Read the model definition and answer for the solid it produces. Units are mm, in the model's axes. Coordinates: 2 decimals unless noted, no trailing zeros. Write each loop counter-clockwise with the first axis right and the second up, starting at its lowest first coordinate (ties: lowest second). Pieces come first, ordered by that corner, then holes.
1) The part is cut by section A-A (z = 1345). Determine the outline of the cut face in (x, y).
2) The part is cut by section D-D (z = 1295.5). Determine the outline of the cut face in (x, y).
3) Find the intervals of material crossed by line 1 (Y direction, x = 29, z = 1343); line 2 (Y direction, x = 28.5, z = 1389); line 3 (Z direction, x = 29.35, y = 236), in increasing order.
4) The part is cut by section B-B (x = 31.2). Give the number of separate pieces and of enclosed holes in the cut face, then the cut area to 3 significant figures.
5) Each of these flat-tipped pins is pushed along its axis until it touches: pin 1 Ø5 at (y, z) = (301.1, 1397.63) entering from +X; pin 2 Ø2 at (x, z) = (29, 1395.5) entering from +Y; pin 3 Ø2 at (x, y) = (30.5, 235.5) entering from -Z. Where does it stop, or does it pass through?
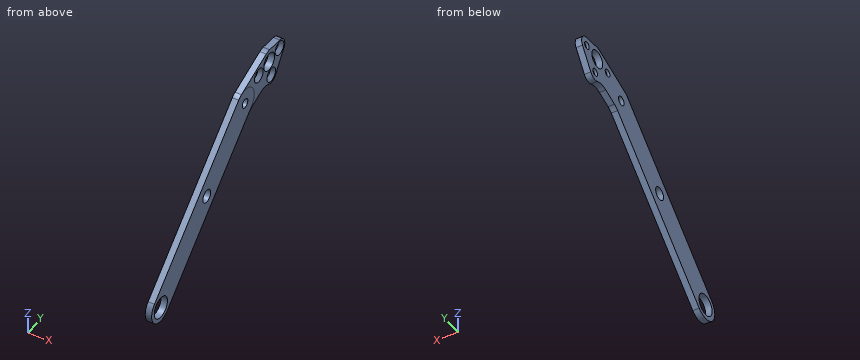
from build123d import *
from OCP.BRepAlgoAPI import BRepAlgoAPI_Cut
from OCP.TopTools import TopTools_ListOfShape

# Parameters (mm, degrees)
BOSS_EXTRUDE1_START                         = 27.641612
SKETCH1_R                                   = 7.9375
BOSS_EXTRUDE1_DEPTH                         = 4.762501
F_1_4_CLEARANCE_HOLE1_D                     = 6.7564
CUT_EXTRUDE1_DEPTH                          = 1429.793432694
CUT_EXTRUDE1_DEPTH_BACK                     = 1429.793432694
SKETCH4_R                                   = 4.7625
BOSS_EXTRUDE2_START                         = 27.641612
BOSS_EXTRUDE2_DEPTH                         = 4.7625
F_1_2_CLEARANCE_HOLE1_D                     = 13.09624
CSK_FOR_10_FLAT_HEAD_SOCKET_CAP_SCR_2_COUNT = 2
CSK_FOR_10_FLAT_HEAD_SOCKET_CAP_SCR_2_PITCH = 17.960512242
CSK_FOR_10_FLAT_HEAD_SOCKET_CAP_SCR_3_COUNT = 2
CSK_FOR_10_FLAT_HEAD_SOCKET_CAP_SCR_3_PITCH = 25.4
FILLET1_R                                   = 12.7


with BuildPart() as part:
    # Sketch1 → Boss-Extrude1 (new body)
    with BuildSketch(Plane(origin=(0, 0, 0), x_dir=(0, 0, -1), z_dir=(1, 0, 0)).offset(BOSS_EXTRUDE1_START)):
        with BuildLine():
            Line((-1394.467062617, 276.836816997), (-1298.446828577, 175.366601392))
            ThreePointArc((-1298.446828577, 175.366601392), (-1282.737360992, 174.933080131), (-1282.303839731, 190.642547716))
            Line((-1282.303839731, 190.642547716), (-1378.32407377, 292.112763322))
            ThreePointArc((-1378.32407377, 292.112763322), (-1394.033541356, 292.546284583), (-1394.467062617, 276.836816997))
        make_face()
        with Locations((-1290.375334154, 183.004574554)):
            Circle(SKETCH1_R, mode=Mode.SUBTRACT)
    extrude(amount=BOSS_EXTRUDE1_DEPTH)

    # 1/4 Clearance Hole1 (through all)
    with Locations(Plane.ZY.offset(-27.641612484)):
        with Locations((1386.395568193, 284.47479016)):
            Hole(F_1_4_CLEARANCE_HOLE1_D / 2)

    # Sketch4 → Cut-Extrude1 (cut, two sides: drawn at the far end of the back side and taken through both)
    with BuildSketch(Plane(origin=(0, 0, 0), x_dir=(0, 0, -1), z_dir=(1, 0, 0)).offset(-CUT_EXTRUDE1_DEPTH_BACK)):
        with Locations((-1342.750007266, 238.351964884)):
            Circle(SKETCH4_R)
    extrude(amount=CUT_EXTRUDE1_DEPTH + CUT_EXTRUDE1_DEPTH_BACK, mode=Mode.SUBTRACT)

    # Sketch5 → Boss-Extrude2 (add)
    with BuildSketch(Plane(origin=(0, 0, 0), x_dir=(0, 0, -1), z_dir=(1, 0, 0)).offset(BOSS_EXTRUDE2_START)):
        with BuildLine():
            Line((-1408.915317884, 326.37077483), (-1409.610698903, 314.093730387))
            ThreePointArc((-1409.610698903, 314.093730387), (-1409.493080384, 311.969736982), (-1408.907003916, 309.924817308))
            Line((-1408.907003916, 309.924817308), (-1396.669308063, 280.239471359))
            ThreePointArc((-1396.669308063, 280.239471359), (-1392.433468222, 293.803853322), (-1378.32407377, 292.112763322))
            Line((-1378.32407377, 292.112763322), (-1376.907390708, 290.615671201))
            Line((-1376.907390708, 290.615671201), (-1385.003560397, 310.254792894))
            ThreePointArc((-1385.003560397, 310.254792894), (-1381.314759969, 315.520916186), (-1384.1151615, 321.308580171))
            Line((-1384.1151615, 321.308580171), (-1399.046290774, 331.290632995))
            ThreePointArc((-1399.046290774, 331.290632995), (-1405.408532388, 331.694665931), (-1408.915317884, 326.37077483))
        make_face()
    extrude(amount=BOSS_EXTRUDE2_DEPTH)

    # 1/2 Clearance Hole1 (through all)
    with Locations(Plane(origin=(32.404112484, 0, 0), x_dir=(0, 0, -1), z_dir=(1, 0, 0))):
        with Locations((-1400.10094117, 313.555090566)):
            Hole(F_1_2_CLEARANCE_HOLE1_D / 2)


with BuildPart() as csk_for_10_flat_head_socket_cap_screw1_tool:
    # Sketch10 → CSK for #10 Flat Head Socket Cap Screw1 (revolve)
    with BuildSketch(Plane(origin=(32.404112484, 326.011681615, 1402.575479395), x_dir=(0, 0, -1), z_dir=(0, 1, 0))):
        Polygon((0, 0), (0, 4.7625), (2.8067, 4.7625), (2.8067, 2.775838967), (5.2197, 0), align=None)
    csk_for_10_flat_head_socket_cap_screw1 = revolve(axis=Axis((38.754112484, 326.011681615, 1402.575479395), (-1, 0, 0)))


with BuildPart() as part_1:
    add(part.part)

    # CSK for #10 Flat Head Socket Cap Screw1: cut by csk_for_10_flat_head_socket_cap_screw1_tool, with a tolerance
    csk_for_10_flat_head_socket_cap_screw1_stock = TopTools_ListOfShape()
    csk_for_10_flat_head_socket_cap_screw1_stock.Append(part_1.part.wrapped)
    csk_for_10_flat_head_socket_cap_screw1_tools = TopTools_ListOfShape()
    csk_for_10_flat_head_socket_cap_screw1_tools.Append(csk_for_10_flat_head_socket_cap_screw1_tool.part.wrapped)
    csk_for_10_flat_head_socket_cap_screw1_cut = BRepAlgoAPI_Cut()
    csk_for_10_flat_head_socket_cap_screw1_cut.SetArguments(csk_for_10_flat_head_socket_cap_screw1_stock)
    csk_for_10_flat_head_socket_cap_screw1_cut.SetTools(csk_for_10_flat_head_socket_cap_screw1_tools)
    csk_for_10_flat_head_socket_cap_screw1_cut.SetFuzzyValue(0.00001)
    csk_for_10_flat_head_socket_cap_screw1_cut.Build()
    add(Compound.cast(csk_for_10_flat_head_socket_cap_screw1_cut.Shape()).solids(), mode=Mode.REPLACE)

    # CSK for _10 Flat Head Socket Cap Scr 2: CSK for #10 Flat Head Socket Cap Screw1 ×2
    with Locations(*[Vector(0, -0.5557777356316841, -0.8313309260313356) * (i * CSK_FOR_10_FLAT_HEAD_SOCKET_CAP_SCR_2_PITCH) for i in range(1, CSK_FOR_10_FLAT_HEAD_SOCKET_CAP_SCR_2_COUNT)]):
        add(csk_for_10_flat_head_socket_cap_screw1, mode=Mode.SUBTRACT)

    # CSK for _10 Flat Head Socket Cap Scr 3: CSK for #10 Flat Head Socket Cap Screw1 ×2
    with Locations(*[Vector(0, -0.9808339409045171, -0.19484552950918363) * (i * CSK_FOR_10_FLAT_HEAD_SOCKET_CAP_SCR_3_PITCH) for i in range(1, CSK_FOR_10_FLAT_HEAD_SOCKET_CAP_SCR_3_COUNT)]):
        add(csk_for_10_flat_head_socket_cap_screw1, mode=Mode.SUBTRACT)

    # Fillet1
    fillet1_edges = [part_1.edges().sort_by_distance(p)[0] for p in [
        (30.022862, 290.615671201, 1376.907390708),
        (30.022862, 310.254792894, 1385.003560397),
    ]]
    fillet(fillet1_edges, radius=FILLET1_R)


solid = part_1.part
Reported:
1. outline: (27.64, 224.56) - (32.4, 224.56) - (32.4, 234.15) - (27.64, 234.15) - close; (27.64, 242.55) - (32.4, 242.55) - (32.4, 256.9) - (27.64, 256.9) - close
2. outline: (27.64, 173.14) - (32.4, 173.14) - (32.4, 176.94) - (27.64, 176.94) - close; (27.64, 189.07) - (32.4, 189.07) - (32.4, 204.59) - (27.64, 204.59) - close
3. line 1: y = 222.45 to 233.6, 243.11 to 254.78
3. line 2: y = 271.06 to 282.32, 286.63 to 313.57, 318.49 to 324.57
3. line 3: z = 1325.23 to 1338.61, 1346.89 to 1355.82
4. separate pieces: 1
4. enclosed holes: 7
4. area: 3,800 mm2
5. pin 1: passes through
5. pin 2: stops at y = 329.59
5. pin 3: stops at z = 1323.81
